Check sheet for the drawn part. Datum: minimum x, y, z corner. Units: mm. Give positions to 0.01 mm unless a question says otherwise; leave off trailing zeros. Loops run counter-clockwise (first coordinate to the right, second up) from the corner with the lowest first, then second, coordinate; pieces in that order, holes last. Notation, with made-up numbers: (48, 28.5) - (62, 28.5) arc R27 ccw to (62, 45.5) - close; hole circle Ø11 at (39, 82). An arc over 180 degrees is marked (long way). Answer in a Markdown table with one row per item.
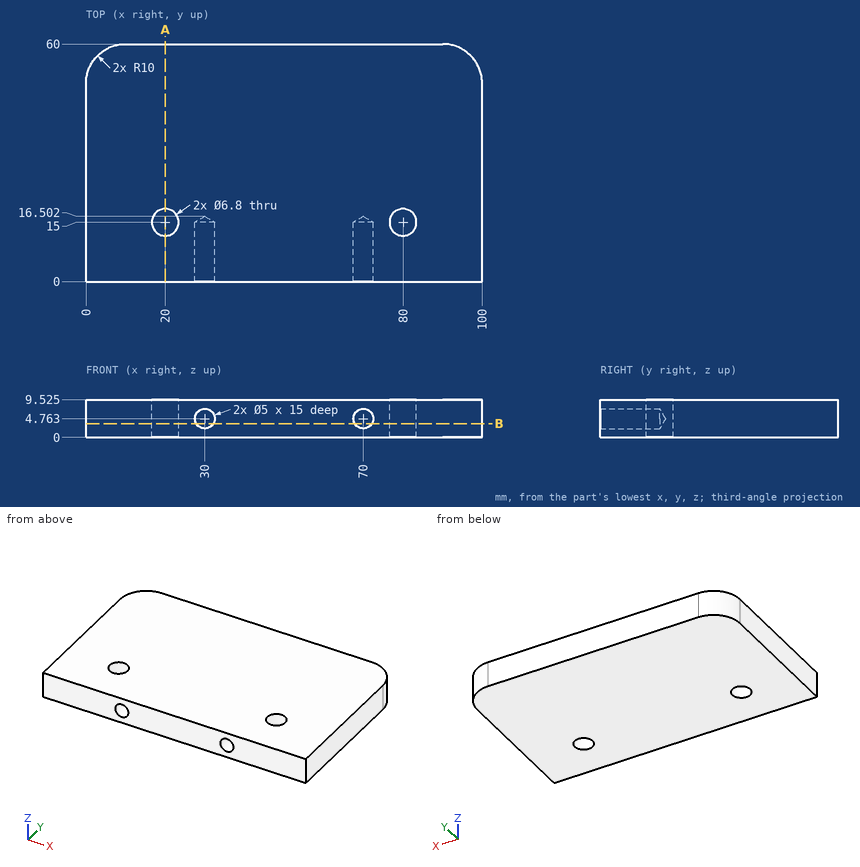
Q1. Sectioned sample at B-B (z = 3.5). Give the number of separate pieces and of enclosed holes in the cut face, and give its area (3 significant figures).
Completed:
| item | result |
|---|---|
| separate pieces | 1 |
| enclosed holes | 2 |
| area | 5,750 mm^2 |
Q2. Go/stop test with a flat-tipped pin: P1, Ø3, axis at x = 70, z = 4.76, coming from the -Y side. Record where the tip stops, or that it passes through.
Completed:
| item | result |
|---|---|
| P1 | y = 15.6 |
Q3. Thickness scan on line 1 (Y direction, x = 20, z = 5.5); line 2 (Z direction, x = 30, y = 8) (1 decimal); line 3 (X direction, y = 17, z = 4.5). Record the ranges inside material, lowest first.
Completed:
| item | result |
|---|---|
| line 1 | 0 to 11.6, 18.4 to 60 |
| line 2 | 0 to 2.3, 7.3 to 9.5 |
| line 3 | 0 to 17.25, 22.75 to 77.25, 82.75 to 100 |
Q4. Sectioned sample at A-A (x = 20). Record the cut outline in (y, z) (1 decimal).
Completed:
| item | result |
|---|---|
| outline | (0, 0) - (11.6, 0) - (11.6, 9.5) - (0, 9.5) - close; (18.4, 0) - (60, 0) - (60, 9.5) - (18.4, 9.5) - close |
